from build123d import *

# Parameters (mm, degrees)
SKETCH1_R           = 9.906
SKETCH1_R_2         = 12.7
BOSS_EXTRUDE1_DEPTH = 5.6896


with BuildPart() as part:
    # Sketch1 → Boss-Extrude1 (new body)
    with BuildSketch(Plane.XY):
        with BuildLine():
            ThreePointArc((-13.085798561, 50.8), (0, 63.885798561), (13.085798561, 50.8))
            Line((13.085798561, 50.8), (15.879798561, 0))
            ThreePointArc((15.879798561, 0), (0, -16.777187541), (-15.879798561, 0))
            Line((-15.879798561, 0), (-13.085798561, 50.8))
        make_face()
        with Locations((0, 50.8)):
            Circle(SKETCH1_R, mode=Mode.SUBTRACT)
        Circle(SKETCH1_R_2, mode=Mode.SUBTRACT)
    extrude(amount=BOSS_EXTRUDE1_DEPTH)


solid = part.part
Can you work these out from the model? Positions are in its coordinate system, mm. Give positions to 0.01 mm unless a question says otherwise; leave off trailing zeros. Loops run counter-clockwise (first coordinate to the right, second up) from the corner with the lowest first, then second, coordinate; pieces in that order, holes last. Notation, with made-up numbers: (30.5, -17.5) -> (39.5, -17.5) arc R22 cw to (39.5, -11.5) -> close; hole circle Ø3 at (11.25, -35.5). An arc over 180 degrees is marked (long way). Write item = value, one per line.
1) Will these pins go through, and if not, where does the flat tip stop? pin 1 (1.5 mm diameter, centred on x = -1, z = 4, fed in from -Y); pin 2 (2 mm diameter, centred on x = -6.5, z = 3.5, fed in from +Y).
Check result:
pin_1 = -16.78
pin_2 = 62.67
2) Suppose I cut it at A-A on x = 0. Write out the boundary of the cut face in (y, z), then the cut area to 3 significant figures.
Check result:
outline = (-16.78, 0) -> (-12.7, 0) -> (-12.7, 5.69) -> (-16.78, 5.69) -> close; (12.7, 0) -> (40.89, 0) -> (40.89, 5.69) -> (12.7, 5.69) -> close; (60.71, 0) -> (63.89, 0) -> (63.89, 5.69) -> (60.71, 5.69) -> close
area = 202 mm2
3) Suppose I cut it at C-C on y = 52. Write out the boundary of the cut face in (x, z).
Check result:
outline = (-13.03, 0) -> (-9.83, 0) -> (-9.83, 5.69) -> (-13.03, 5.69) -> close; (9.83, 0) -> (13.03, 0) -> (13.03, 5.69) -> (9.83, 5.69) -> close
4) Thinking about a two-plate mould opening in Y: for faces 1 (the flat face through (0, 24, 5.69)), 2 (the cylindrical face through (-2.75, -12.4, 2.8)), 3 (the flat face through (-14.502, 25.044, 2.805)), which applies, released by +Y, released by -Y, zero draft, split by the parting line, or undercut?
Check result:
face_1 = zero draft
face_2 = undercut
face_3 = released by +Y
5) Suppose I cut it at B-B on z = 3.45. Write out the boundary of the cut face in (x, y).
Check result:
outline = (-15.88, 0) arc R15.9 ccw (long way) to (15.88, 0) -> (13.09, 50.8) arc R13.09 ccw to (-13.09, 50.8) -> close; hole circle Ø25.4 at (0, 0); hole circle Ø19.81 at (0, 50.8)
6) Suppose I cut it at D-D on x = 12. Write out the boundary of the cut face in (y, z).
Check result:
outline = (-11.31, 0) -> (-4.16, 0) -> (-4.16, 5.69) -> (-11.31, 5.69) -> close; (4.16, 0) -> (56.02, 0) -> (56.02, 5.69) -> (4.16, 5.69) -> close
7) I need wall thicknesses on L1, parallel to Y at x = 0, z = 2.5; L2, parallel to Y at x = -7.5, z = 3.55; L3, parallel to X at y = -1.5, z = 4.35. Which ranges of each line are inside material? Lowest first, please. Write a range as from..to.
Check result:
L1 = -16.78..-12.7, 12.7..40.89, 60.71..63.89
L2 = -14.9..-10.25, 10.25..44.33, 57.27..61.52
L3 = -15.89..-12.61, 12.61..15.89
